```python
from build123d import *

# Parameters (mm, degrees)
F1_DEPTH = 25


with BuildPart() as f1:
    # F0 (on Front) → F1 (new body)
    with BuildSketch(Plane.XZ):
        with BuildLine():
            ThreePointArc((-4.330127, 2.5), (0, 5), (4.330127, 2.5))
            Line((4.330127, 2.5), (9.682458, 2.5))
            ThreePointArc((9.682458, 2.5), (6.123724, 7.905694), (0, 10))
            ThreePointArc((0, 10), (-6.123724, 7.905694), (-9.682458, 2.5))
            Line((-9.682458, 2.5), (-4.330127, 2.5))
        make_face()
        with BuildLine():
            ThreePointArc((4.330127, 2.5), (4.829629, 1.294095), (5, 0))
            ThreePointArc((5, 0), (4.829629, -1.294095), (4.330127, -2.5))
            Line((4.330127, -2.5), (9.682458, -2.5))
            Line((9.682458, -2.5), (19.330127, -2.5))
            Line((19.330127, -2.5), (19.330127, 2.5))
            Line((19.330127, 2.5), (9.682458, 2.5))
            Line((9.682458, 2.5), (4.330127, 2.5))
        make_face()
        with BuildLine():
            Line((9.682458, -2.5), (4.330127, -2.5))
            ThreePointArc((4.330127, -2.5), (0, -5), (-4.330127, -2.5))
            Line((-4.330127, -2.5), (-9.682458, -2.5))
            ThreePointArc((-9.682458, -2.5), (-6.123724, -7.905694), (0, -10))
            ThreePointArc((0, -10), (6.123724, -7.905694), (9.682458, -2.5))
        make_face()
        with BuildLine():
            ThreePointArc((-4.330127, -2.5), (-5, 0), (-4.330127, 2.5))
            Line((-4.330127, 2.5), (-9.682458, 2.5))
            ThreePointArc((-9.682458, 2.5), (-10, 0), (-9.682458, -2.5))
            Line((-9.682458, -2.5), (-4.330127, -2.5))
        make_face()
        with BuildLine():
            ThreePointArc((0, 10), (6.123724, 7.905694), (9.682458, 2.5))
            Line((9.682458, 2.5), (19.330127, 2.5))
            Line((19.330127, 2.5), (19.330127, 5))
            Line((19.330127, 5), (15, 10))
            Line((15, 10), (0, 10))
        make_face()
        with BuildLine():
            Line((19.330127, -2.5), (9.682458, -2.5))
            ThreePointArc((9.682458, -2.5), (6.123724, -7.905694), (0, -10))
            Line((0, -10), (15, -10))
            Line((15, -10), (19.330127, -5))
            Line((19.330127, -5), (19.330127, -2.5))
        make_face()
    extrude(amount=F1_DEPTH)


solid = f1.part
```
CAD build for the part. Positions are in the model's coordinates, mm. Round coordinates to 2 decimals unless told otherwise and drop trailing zeros. Write each loop counter-clockwise with the first axis right and the second up, starting at its lowest first coordinate (ties: lowest second). Pieces come first, ordered by that corner, then holes. Notation, with made-up numbers: (-15, 45) - (-11, 45) arc R17 ccw to (-11, 68) - close; hole circle Ø4 at (52.5, 57). An arc over 180 degrees is marked (long way). Return JSON: item names as keys, results as strings. Group by question number.
Item 1: Flat gauge pins, fed straight in: pin 1 Ø2 at (y, z) = (-12, 5) entering from -X; pin 2 Ø5 at (y, z) = (-4, -5) entering from -X; pin 3 Ø1 at (x, y) = (-3, -10) entering from +Z. Where does each tip first touch, or does it go through?
Item 2: Band-saw the part on D-D on x = 16.25. List the corners of the cut face in (y, z).
Item 3: Band-saw the part on B-B on x = 1. List the corners of the cut face in (y, z).
Item 4: Band-saw the part on C-C on z = 0.5. List the corners of the cut face in (x, y), plus the area to 3 significant figures.
Item 5: Probe probe 1 along Z at (x, y) = (2.5, -21.5); probe 2 along Z at (x, y) = (-4.5, -14); probe 3 along X at (y, z) = (-15.25, 3). List the from-to ranges inside material, lowest first.
Item 6: Band-saw the part on A-A on y = -14.25. List the corners of the cut face in (x, z), plus the area to 3 significant figures.
Resolved:
{
 "1": {"pin 1": "stops at x = -9.17", "pin 2": "stops at x = -9.68", "pin 3": "stops at z = 9.68"},
 "2": {"outline": "(-25, -8.56) - (0, -8.56) - (0, 8.56) - (-25, 8.56) - close"},
 "3": {"outline": "(-25, -10) - (0, -10) - (0, -4.9) - (-25, -4.9) - close; (-25, 4.9) - (0, 4.9) - (0, 10) - (-25, 10) - close"},
 "4": {"outline": "(-9.99, -25) - (-4.97, -25) - (-4.97, 0) - (-9.99, 0) - close; (4.97, -25) - (19.33, -25) - (19.33, 0) - (4.97, 0) - close", "area": "484 mm²"},
 "5": {"probe 1": "z = -10 to -4.33, 4.33 to 10", "probe 2": "z = -8.93 to -2.18, 2.18 to 8.93", "probe 3": "x = -9.54 to -4, 4 to 19.33"},
 "6": {"outline": "(-9.68, -2.5) arc R10 ccw to (0, -10) - (15, -10) - (19.33, -5) - (19.33, 5) - (15, 10) - (0, 10) arc R10 ccw to (-9.68, 2.5) arc R10 ccw to start; hole (4.33, -2.5) arc R5 ccw to (5, 0) arc R5 ccw to (4.33, 2.5) arc R5 ccw (long way) to start", "area": "443 mm²"}
}
